from build123d import *

# Parameters (mm, degrees)
F1_DEPTH = 10
F3_DEPTH = 10.001
F4_R     = 3


with BuildPart() as f1:
    # F0 (on Top) → F1 (new body)
    with BuildSketch(Plane.XY):
        with BuildLine():
            ThreePointArc((8.269933, 4.774648), (6.943567, 12.026611), (0, 9.549297))
            ThreePointArc((0, 9.549297), (0.313189, 7.836921), (0, 6.124545))
            ThreePointArc((0, 6.124545), (-3.745285, 3.062272), (-8.269933, 4.774648))
            ThreePointArc((-8.269933, 4.774648), (-13.887134, 0), (-8.269933, -4.774648))
            ThreePointArc((-8.269933, -4.774648), (-2.105729, -3.64723), (0, -9.549297))
            ThreePointArc((0, -9.549297), (6.943567, -12.026611), (8.269933, -4.774648))
            ThreePointArc((8.269933, -4.774648), (4.211459, 0), (8.269933, 4.774648))
        make_face()
    extrude(amount=F1_DEPTH)

    # F2 (on face) → F3 (cut, through all)
    with BuildSketch(Plane.XY.offset(10)):
        with BuildLine():
            Line((-1.65, 1.878164), (-1.65, -1.878164))
            ThreePointArc((-1.65, -1.878164), (0, -2.5), (1.65, -1.878164))
            Line((1.65, -1.878164), (1.65, 1.878164))
            ThreePointArc((1.65, 1.878164), (0, 2.5), (-1.65, 1.878164))
        make_face()
    extrude(amount=-F3_DEPTH, mode=Mode.SUBTRACT)

    # F4
    f4_edges = [f1.edges().sort_by_distance(p)[0] for p in [
        (0, 9.549297, 5),
        (8.269933, 4.774648, 5),
        (8.269933, -4.774648, 5),
        (-8.269933, -4.774648, 5),
        (-8.269933, 4.774648, 5),
        (0, -9.549297, 5),
    ]]
    fillet(f4_edges, radius=F4_R)


solid = f1.part
Check sheet for the modelled part. Datum: model origin and axes. Units: mm. A direction names the side the tool comes from. Give positions to 0.01 mm unless a question says otherwise; leave off trailing zeros. Loops run counter-clockwise (first coordinate to the right, second up) from the corner with the lowest first, then second, coordinate; pieces in that order, holes last. Notation, with made-up numbers: M -40,3.25 L 11,3.25 A13 cw 11,24.25 Z; hole C 46.25,12.5 d3. An arc over 180 degrees is marked long. Return JSON: item names as keys, results as strings. Group by question number.
1. Cross-section at A-A on y = -0.5. Record the boundary of the cut face in (x, z), plus the area to 3 significant figures.
2. Cross-section at B-B on x = -3. Record the boundary of the cut face in (y, z).
3. Tool access check on faces 1 (the flat face through (-1.65, 0, 5)), 2 (the cylindrical face through (4.212, -0.082, 4.93)). Record the directions out of +Z, -Z, +X, -X, +Y, -Y that give a thin tool (end or side, any length) a straight path to the whole face; none if there is none.
4. Cross-section at C-C on y = -8. Record the boundary of the cut face in (x, z).
5. Thickness scan on L1, parallel to X at y = -7.75, z = 8.75; L2, parallel to Y at x = 7, z = 9.25; L3, parallel to Y at x = -0.75, z = 7.5. Record the ranges inside material, lowest first.
6. Go/stop test with flat-tipped pins: pin 1 (2 mm diameter, centred on y = 7.5, z = 4.5, fed in from -X); pin 2 (5 mm diameter, centred on x = -0.5, z = 8.5, fed in from -Y); pin 3 (4 mm diameter, centred on y = -0.5, z = 6, fed in from +X). Record where each tip stops, or that it passes through.
7. Mould release check, pull along Y, two halves, no side actions. Record for faces 3 (the flat face through (-2, 0, 10)), 4 (the cylindrical face through (-13.886, 0.09, 4.93)), 5 (the cylindrical face through (0, -2.5, 5.1)): released by +Y, released by -Y, zero draft, split by the parting line, or undercut.
Return value:
{
 "1": {"outline": "M -13.86,0 L -1.65,0 L -1.65,10 L -13.86,10 Z; M 1.65,0 L 4.24,0 L 4.24,10 L 1.65,10 Z", "area": "148 mm^2"},
 "2": {"outline": "M -3.25,0 L 3.25,0 L 3.25,10 L -3.25,10 Z"},
 "3": {"face 1": "+Z, -Z", "face 2": "+Z, -Z, +X"},
 "4": {"outline": "M 0.31,0 L 9.36,0 L 9.36,10 L 0.31,10 Z"},
 "5": {"L1": "0.31 to 9.36", "L2": "-11.99 to -4.38, 4.38 to 11.99", "L3": "-4.81 to -2.38, 2.38 to 4.81"},
 "6": {"pin 1": "x = 0.12", "pin 2": "y = -11.96", "pin 3": "x = 4.91"},
 "7": {"face 3": "zero draft", "face 4": "split by the parting line", "face 5": "undercut"}
}
